```python
from build123d import *

# Parameters (mm, degrees)
SKETCH1_W               = 25
SKETCH1_H               = 480
BOSS_EXTRUDE1_DEPTH     = 50
BOSS_EXTRUDE1_2_DEPTH   = 50
SHELL1_T                = -1.5
SHELL2_T                = -1.5
SKETCH2_W               = 180
SKETCH2_H               = 40
BOSS_EXTRUDE2_DEPTH     = 4
SKETCH3_W               = 180
SKETCH3_H               = 40
BOSS_EXTRUDE3_DEPTH     = 4
CUT_EXTRUDE1_DEPTH      = 1306.595649503
CUT_EXTRUDE1_DEPTH_BACK = 1306.595649503
SKETCH4_R               = 3.5
SKETCH5_R               = 3.5
BOSS_EXTRUDE4_DEPTH     = 25
BOSS_EXTRUDE5_START     = 25
SKETCH6_R               = 3.5
BOSS_EXTRUDE5_DEPTH     = 25
CUT_EXTRUDE6_DEPTH      = 1306.595649503
CUT_EXTRUDE6_DEPTH_BACK = 1306.595649503
CUT_EXTRUDE7_DEPTH      = 1306.595649503
CUT_EXTRUDE7_DEPTH_BACK = 1306.595649503


with BuildPart() as part:
    # Sketch1 → Boss-Extrude1 (new body)
    with BuildSketch(Plane.XY):
        with Locations((-160.684832451, -1052)):
            Rectangle(SKETCH1_W, SKETCH1_H)
    extrude(amount=BOSS_EXTRUDE1_DEPTH)

    # Shell2
    shell2_openings = [part.faces().sort_by_distance(p)[0] for p in [
        (-160.684832451, -1292, 25),
        (-160.684832451, -812, 25),
    ]]
    offset(amount=SHELL2_T, openings=shell2_openings, kind=Kind.INTERSECTION)



with BuildPart() as body_2:
    # Sketch1 → Boss-Extrude1 2 (new body)
    with BuildSketch(Plane.XY):
        with Locations((-315.684832451, -1052)):
            Rectangle(SKETCH1_W, SKETCH1_H)
    extrude(amount=BOSS_EXTRUDE1_2_DEPTH)

    # Shell1
    shell1_openings = [body_2.faces().sort_by_distance(p)[0] for p in [
        (-315.684832451, -812, 25),
        (-315.684832451, -1292, 25),
    ]]
    offset(amount=SHELL1_T, openings=shell1_openings, kind=Kind.INTERSECTION)


with BuildPart() as part_1:
    add(part.part)

    add(body_2.part)  # Boss-Extrude2 merges body 2
    # Sketch2 → Boss-Extrude2 (add)
    with BuildSketch(Plane.XY):
        with Locations((-238.184832451, -1197)):
            Rectangle(SKETCH2_W, SKETCH2_H)
    extrude(amount=BOSS_EXTRUDE2_DEPTH)

    # Sketch3 → Boss-Extrude3 (add)
    with BuildSketch(Plane.XY.offset(50)):
        with Locations((-238.184832451, -907)):
            Rectangle(SKETCH3_W, SKETCH3_H)
    extrude(amount=BOSS_EXTRUDE3_DEPTH)

    # Sketch4 → Cut-Extrude1 (cut, two sides: drawn at the far end of the back side and taken through both)
    with BuildSketch(Plane.ZY.offset(328.184832451).offset(-CUT_EXTRUDE1_DEPTH_BACK)):
        with Locations((25, -1267)):
            Circle(SKETCH4_R)
        with Locations((25, -832)):
            Circle(SKETCH4_R)
    extrude(amount=CUT_EXTRUDE1_DEPTH + CUT_EXTRUDE1_DEPTH_BACK, mode=Mode.SUBTRACT)

    # Sketch5 → Boss-Extrude4 (add)
    with BuildSketch(Plane(origin=(-303.184832451, 0, 0), x_dir=(0, 0, -1), z_dir=(1, 0, 0))):
        with Locations(Location((-25, -1052, 0), (0, 0, 270))):
            Circle(SKETCH5_R)
    extrude(amount=BOSS_EXTRUDE4_DEPTH)

    # Sketch6 → Boss-Extrude5 (add)
    with BuildSketch(Plane.ZY.offset(173.184832451).offset(BOSS_EXTRUDE5_START)):
        with Locations(Location((25, -1052, 0), (0, 0, 270))):
            Circle(SKETCH6_R)
    extrude(amount=-BOSS_EXTRUDE5_DEPTH)

    # Sketch11 → Cut-Extrude6 (cut, two sides: drawn at the far end of the back side and taken through both)
    with BuildSketch(Plane.ZY.offset(328.184832451).offset(-CUT_EXTRUDE6_DEPTH_BACK)):
        Polygon((25, -812), (50, -852.824757881), (50, -812), align=None)
    extrude(amount=CUT_EXTRUDE6_DEPTH + CUT_EXTRUDE6_DEPTH_BACK, mode=Mode.SUBTRACT)

    # Sketch12 → Cut-Extrude7 (cut, two sides: drawn at the far end of the back side and taken through both)
    with BuildSketch(Plane.ZY.offset(328.184832451).offset(-CUT_EXTRUDE7_DEPTH_BACK)):
        Polygon((25, -1292), (0, -1241.284902425), (0, -1292), align=None)
    extrude(amount=CUT_EXTRUDE7_DEPTH + CUT_EXTRUDE7_DEPTH_BACK, mode=Mode.SUBTRACT)


solid = part_1.part
```
The listing builds one solid part. Answer for the finished solid, in the listing's coordinates (mm). A direction names the side the tool comes from. Coordinates: 2 decimals unless noted, no trailing zeros. Write each loop counter-clockwise with the first axis right and the second up, starting at its lowest first coordinate (ties: lowest second). Pieces come first, ordered by that corner, then holes. Notation, with made-up numbers: (23.5, 56) - (73.5, 56) arc R24 ccw to (73.5, 69) - close; hole circle Ø5 at (-39, 7). An arc over 180 degrees is marked (long way). One line per item, written item: value.
1) A tool of negligible diameter and unlimited length cuts with its end or side. For faces 1 (the flat face through (-316, -870, 50)), 2 (the flat face through (-316, -1197, 4)), 3 (the flat face through (-316, -1230, 1.5)), 4 (the flat face through (-239, -907, 50)), from which of +Z, -Z, +X, -X, +Y, -Y can it reach the whole face along a straight path? Write none if from no direction.
Geometry check:
face 1: +Z, +X, -X, +Y
face 2: +Y, -Y
face 3: -Y
face 4: -Z, +Y, -Y
2) Each of these flat-tipped pins is pushed along its axis until it touches: pin 1 Ø5 at (x, y) = (-258.5, -1212) entering from +Z; pin 2 Ø10 at (x, z) = (-202, 28) entering from +Y; pin 3 Ø17.5 at (x, y) = (-160.5, -1234) entering from +Z. Where does it stop, or does it pass through?
Geometry check:
pin 1: stops at z = 4
pin 2: stops at y = -1048.5
pin 3: stops at z = 50
3) Consider line 1 along X through (y, z) = (-1220.5, 12); line 2 along Y through (x, z) = (-303.75, 25); line 3 along Z through (x, y) = (-156.5, -1148). Determine where each line is inside the solid, lowest interval first. Write a range as from..to.
Geometry check:
line 1: x = -328.18..-326.68, -304.68..-303.18, -173.18..-171.68, -149.68..-148.18
line 2: y = -1292..-1270.5, -1263.5..-835.5, -828.5..-812
line 3: z = 0..1.5, 48.5..50
4) For a pull along Z with two mould halves and no side action, classify faces 5 (the flat face through (-316, -1107, 50)), 6 (the flat face through (-171.685, -1055, 25)), 7 (the flat face through (-316, -1292, 49)), 8 (the flat face through (-161, -1197, 4)) as pulls with the +Z half, pulls with the -Z half, needs draft (parallel to the pull), parting line crosses it, or undercut.
Geometry check:
face 5: pulls with the +Z half
face 6: undercut
face 7: needs draft
face 8: undercut
5) Find section B-B (z = 39). Give the vertices of the cut face in (x, y), and give its area (3 significant figures).
Geometry check:
outline: (-328.18, -1292) - (-326.68, -1292) - (-326.68, -834.86) - (-328.18, -834.86) - close; (-304.68, -1292) - (-303.18, -1292) - (-303.18, -834.86) - (-304.68, -834.86) - close; (-173.18, -1292) - (-171.68, -1292) - (-171.68, -834.86) - (-173.18, -834.86) - close; (-149.68, -1292) - (-148.18, -1292) - (-148.18, -834.86) - (-149.68, -834.86) - close
area: 2,740 mm2
6) Find section D-D (x = -224). Give the vertices of the cut face in (y, z).
Geometry check:
outline: (-1217, 0) - (-1177, 0) - (-1177, 4) - (-1217, 4) - close; (-927, 50) - (-887, 50) - (-887, 54) - (-927, 54) - close
7) Find section C-C (y = -912.5). Give the vertices of the cut face in (x, z).
Geometry check:
outline: (-328.18, 0) - (-303.18, 0) - (-303.18, 50) - (-173.18, 50) - (-173.18, 0) - (-148.18, 0) - (-148.18, 54) - (-328.18, 54) - close; hole (-326.68, 1.5) - (-304.68, 1.5) - (-304.68, 48.5) - (-326.68, 48.5) - close; hole (-171.68, 1.5) - (-149.68, 1.5) - (-149.68, 48.5) - (-171.68, 48.5) - close
8) Find section A-A (x = -184). Give the vertices of the cut face in (y, z), and give its area (3 significant figures).
Geometry check:
outline: (-1217, 0) - (-1177, 0) - (-1177, 4) - (-1217, 4) - close; circle Ø7 at (-1052, 25); (-927, 50) - (-887, 50) - (-887, 54) - (-927, 54) - close
area: 358 mm2
